from build123d import *

# Parameters (mm, degrees)
BOSS_EXTRUDE1_DEPTH = 20.9
CUT_EXTRUDE1_DEPTH  = 57.895670946
SKETCH4_R           = 2.5
CUT_EXTRUDE2_DEPTH  = 57.389876565
SKETCH5_R           = 4.2
SKETCH5_R_2         = 2.5
BOSS_EXTRUDE2_DEPTH = 2
FILLET1_R           = 0.6


with BuildPart() as part:
    # Sketch1 → Boss-Extrude1 (new body)
    with BuildSketch(Plane.XY):
        with BuildLine():
            Line((1.6, 0), (1.6, 11.647897552))
            ThreePointArc((1.6, 11.647897552), (1.793345987, 12.61991347), (2.343948776, 13.443948776))
            Line((2.343948776, 13.443948776), (9.836307345, 20.936307345))
            ThreePointArc((9.836307345, 20.936307345), (10.386910134, 21.760342651), (10.580256121, 22.732358569))
            Line((10.580256121, 22.732358569), (10.580256121, 33.328153673))
            ThreePointArc((10.580256121, 33.328153673), (10.773602108, 34.300169591), (11.324204897, 35.124204897))
            Line((11.324204897, 35.124204897), (24.948665915, 48.748665915))
            Line((24.948665915, 48.748665915), (23.817295065, 49.880036765))
            Line((23.817295065, 49.880036765), (9.724204897, 35.786946597))
            ThreePointArc((9.724204897, 35.786946597), (9.173602108, 34.962911291), (8.980256121, 33.990895372))
            Line((8.980256121, 33.990895372), (8.980256121, 23.395100269))
            ThreePointArc((8.980256121, 23.395100269), (8.786910134, 22.423084351), (8.236307345, 21.599049045))
            Line((8.236307345, 21.599049045), (0.743948776, 14.106690476))
            ThreePointArc((0.743948776, 14.106690476), (0.193345987, 13.28265517), (0, 12.310639251))
            Line((0, 12.310639251), (0, 0))
            Line((0, 0), (1.6, 0))
        make_face()
    extrude(amount=-BOSS_EXTRUDE1_DEPTH)

    # Sketch3 → Cut-Extrude1 (cut, through all)
    with BuildSketch(Plane(origin=(-13.03137085, 13.03137085, 0), x_dir=(0, 0, 1), z_dir=(-0.7071067811865472, 0.7071067811865479, 0))):
        with BuildLine():
            ThreePointArc((-20.9, 41.661883092), (-17.839265863, 49.051148955), (-10.45, 52.111883092))
            Line((-10.45, 52.111883092), (-20.9, 52.111883092))
            Line((-20.9, 52.111883092), (-20.9, 41.661883092))
        make_face()
        with BuildLine():
            ThreePointArc((-10.45, 52.111883092), (-3.060734137, 49.051148955), (0, 41.661883092))
            Line((0, 41.661883092), (0, 52.111883092))
            Line((0, 52.111883092), (-10.45, 52.111883092))
        make_face()
    extrude(amount=-CUT_EXTRUDE1_DEPTH, mode=Mode.SUBTRACT)

    # Sketch4 → Cut-Extrude2 (cut, through all)
    with BuildSketch(Plane.ZY.offset(-8.980256121)):
        with Locations(Location((-10.45, 28.692997821, 0), (0, 0, 270))):
            Circle(SKETCH4_R)
    extrude(amount=-CUT_EXTRUDE2_DEPTH, mode=Mode.SUBTRACT)

    # Sketch5 → Boss-Extrude2 (add)
    with BuildSketch(Plane(origin=(10.580256121, 0, 0), x_dir=(0, 0, -1), z_dir=(1, 0, 0))):
        with Locations(Location((10.45, 28.692997821, 0), (0, 0, 90))):
            Circle(SKETCH5_R)
        with Locations(Location((10.45, 28.692997821, 0), (0, 0, 270))):
            Circle(SKETCH5_R_2, mode=Mode.SUBTRACT)
    extrude(amount=BOSS_EXTRUDE2_DEPTH)

    # Fillet1
    fillet1_edges = [part.edges().sort_by_distance(p)[0] for p in [
        (8.980256121, 31.192997821, -10.45),
        (10.580256121, 24.492997821, -10.45),
    ]]
    fillet(fillet1_edges, radius=FILLET1_R)


solid = part.part
Check sheet for the modelled part. Datum: model origin and axes. Units: mm. A direction names the side the tool comes from. Give positions to 0.01 mm unless a question says otherwise; leave off trailing zeros. Loops run counter-clockwise (first coordinate to the right, second up) from the corner with the lowest first, then second, coordinate; pieces in that order, holes last. Notation, with made-up numbers: M 68,40 L 126,40 A14 ccw 126,55 Z; hole C -20.5,66.5 d2. An arc over 180 degrees is marked long. Return JSON: item names as keys, results as strings. Group by question number.
1. Thickness scan on L1, parallel to Y at x = 11.4, z = -10.45; L2, parallel to X at y = 11, z = -0.75; L3, parallel to Y at x = 10.35, z = -10.45. Record the ranges inside material, lowest first.
2. Tool access check on faces 4 (the flat face through (1, 0, -10)), 5 (the flat face through (1.6, 6, -10)), 6 (the cylindrical face through (11.87, 32.7, -9.19)). Record the directions out of +Z, -Z, +X, -X, +Y, -Y that give a thin tool (end or side, any length) a straight path to the whole face; none if there is none.
3. Cross-section at C-C on z = -4. Record the boundary of the cut face in (x, y).
4. Cross-section at A-A on z = -17.25. Record the boundary of the cut face in (x, y), plus the area to 3 significant figures.
5. Go/stop test with flat-tipped pins: pin 1 (10 mm diameter, centred on y = 24.5, z = -17, fed in from -X); pin 2 (6.5 mm diameter, centred on y = 28.69, z = -10.45, fed in from -X); pin 3 (4 mm diameter, centred on x = 10.5, z = -15, fed in from +Y); pin 4 (6 mm diameter, centred on x = 22.5, z = -13, fed in from +Y). Record where each tip stops, or that it passes through.
6. Mould release check, pull along Y, two halves, no side actions. Record for faces 1 (the flat face through (8.98, 31, -13)), 2 (the cylindrical face through (11.06, 31.19, -10.56)), 3 (the flat face through (6, 17.1, -10.3)): released by +Y, released by -Y, zero draft, split by the parting line, or undercut.
7. Cross-section at B-B on y = 6. Record the boundary of the cut face in (x, z), plus the area to 3 significant figures.
Return value:
{
 "1": {"L1": "24.49 to 26.19, 31.19 to 32.89, 35.2 to 37.46", "L2": "0 to 1.6", "L3": "21.68 to 26.19, 31.19 to 36.41"},
 "2": {"face 4": "+Z, -Z, +X, -X, -Y", "face 5": "+Z, -Z, +X, -Y", "face 6": "+X"},
 "3": {"outline": "M 0,0 L 1.6,0 L 1.6,11.65 A2.54 cw 2.34,13.44 L 9.84,20.94 A2.54 ccw 10.58,22.73 L 10.58,33.33 A2.54 cw 11.32,35.12 L 23.37,47.17 L 22.24,48.3 L 9.72,35.79 A2.54 ccw 8.98,33.99 L 8.98,23.4 A2.54 cw 8.24,21.6 L 0.74,14.11 A2.54 ccw 0,12.31 Z"},
 "4": {"outline": "M 0,0 L 1.6,0 L 1.6,11.65 A2.54 cw 2.34,13.44 L 9.84,20.94 A2.54 ccw 10.58,22.73 L 10.58,33.33 A2.54 cw 11.32,35.12 L 23.17,46.97 L 22.04,48.1 L 9.72,35.79 A2.54 ccw 8.98,33.99 L 8.98,23.4 A2.54 cw 8.24,21.6 L 0.74,14.11 A2.54 ccw 0,12.31 Z", "area": "90.5 mm^2"},
 "5": {"pin 1": "x = 6.14", "pin 2": "x = 8.98", "pin 3": "y = 38.56", "pin 4": "y = 49.88"},
 "6": {"face 1": "zero draft", "face 2": "undercut", "face 3": "released by -Y"},
 "7": {"outline": "M 0,-20.9 L 1.6,-20.9 L 1.6,0 L 0,0 Z", "area": "33.4 mm^2"}
}
